Study the drawing (mm; zero at the part's minimum x, y, z) and answer. Coordinates: 2 decimals unless noted, no trailing zeros. Order: outer loops, then holes, each group sorted by start corner. A loop starts at its lowest first (then second) coordinate and runs counter-clockwise, first axis right, second up.
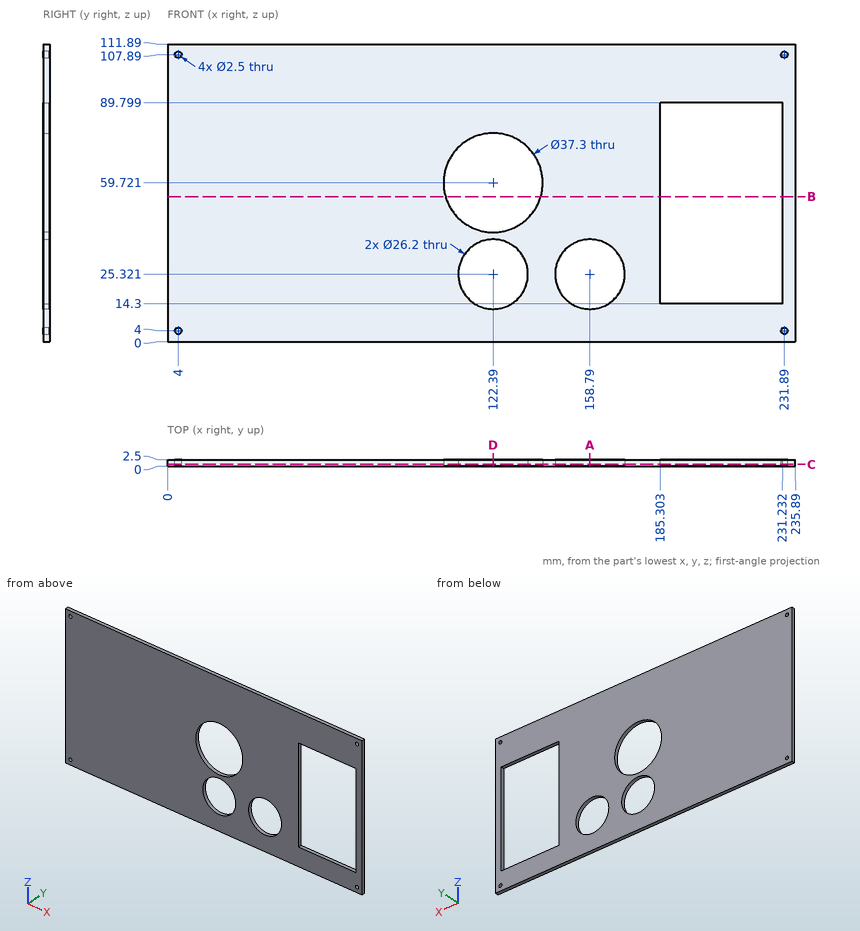
(1) Find section B-B (z = 54.5). Write down the section's boundary in (x, y).
(2) Find section C-C (y = 0.7). Give the number of separate pieces and of enclosed holes in the cut face, and give its area (3 significant figures).
(3) Find section A-A (x = 158.79). Write down the section's boundary in (y, z), and give its area (3 significant figures).
(4) Find section D-D (x = 122.39). Write down the section's boundary in (y, z).
(5) Consider line 1 (X direction, y = 0.65, z = 107.89); line 2 (Z direction, x = 4, y = 1.65); line 3 (Z direction, x = 122.39, y = 1.3). Determine where each line is inside the solid, lowest interval first.
(6) This flat-tipped pin is pushed along its axis until it touches: pin 1 Ø3 at (x, z) = (4, 107.89) entering from +Y. Where does it stop, or does it pass through?
Findings below:
1. outline: (0, 0) - (104.49, 0) - (104.49, 2.5) - (0, 2.5) - close; (140.29, 0) - (185.3, 0) - (185.3, 2.5) - (140.29, 2.5) - close; (231.23, 0) - (235.89, 0) - (235.89, 2.5) - (231.23, 2.5) - close
2. separate pieces: 1
2. enclosed holes: 8
2. area: 20,700 mm2
3. outline: (0, 0) - (2.5, 0) - (2.5, 12.22) - (0, 12.22) - close; (0, 38.42) - (2.5, 38.42) - (2.5, 111.89) - (0, 111.89) - close
3. area: 214 mm2
4. outline: (0, 0) - (2.5, 0) - (2.5, 12.22) - (0, 12.22) - close; (0, 38.42) - (2.5, 38.42) - (2.5, 41.07) - (0, 41.07) - close; (0, 78.37) - (2.5, 78.37) - (2.5, 111.89) - (0, 111.89) - close
5. line 1: x = 0 to 2.75, 5.25 to 230.64, 233.14 to 235.89
5. line 2: z = 0 to 2.75, 5.25 to 106.64, 109.14 to 111.89
5. line 3: z = 0 to 12.22, 38.42 to 41.07, 78.37 to 111.89
6. pin 1: stops at y = 2.5
